For this review, take the finished solid that the model builds, in its own axes (mm). A direction names the side the tool comes from. Round coordinates to 2 decimals unless told otherwise and drop trailing zeros. Loops run counter-clockwise (first coordinate to the right, second up) from the corner with the lowest first, then second, coordinate; pieces in that order, holes last. Notation, with made-up numbers: M 75.5,6 L 112.5,6 A19 ccw 112.5,34 Z; hole C 76,0 d2. An arc over 180 degrees is marked long. Write item = value, one per line. Start each with the question number.
```python
from build123d import *

# Parameters (mm, degrees)
SKETCH1_W           = 118.75
SKETCH1_H           = 24
BOSS_EXTRUDE1_DEPTH = 10
SKETCH2_W           = 3.3
SKETCH2_H           = 9.8
BOSS_EXTRUDE2_DEPTH = 118.75
SKETCH3_W           = 3.3
SKETCH3_H           = 33.8
BOSS_EXTRUDE3_DEPTH = 4.9
CUT_EXTRUDE1_REACH  = 123.333
SKETCH4_R           = 1.9
LPATTERN1_COUNT     = 5
LPATTERN1_PITCH     = 23.75


with BuildPart() as part:
    # Sketch1 → Boss-Extrude1 (new body)
    with BuildSketch(Plane.YZ):
        with Locations((59.375, 12)):
            Rectangle(SKETCH1_W, SKETCH1_H)
    extrude(amount=-BOSS_EXTRUDE1_DEPTH)

    # Sketch2 → Boss-Extrude2 (add, through all)
    with BuildSketch(Plane.XZ):
        with Locations((-5, -4.9)):
            Rectangle(SKETCH2_W, SKETCH2_H)
    extrude(amount=-BOSS_EXTRUDE2_DEPTH)

    # Sketch3 → Boss-Extrude3 (add)
    with BuildSketch(Plane.XZ):
        with Locations((-5, 7.1)):
            Rectangle(SKETCH3_W, SKETCH3_H)
    extrude(amount=BOSS_EXTRUDE3_DEPTH)

    # Sketch4 → Cut-Extrude1 (cut, up to next)
    with BuildSketch(Plane(origin=(-6.65, 0, 0), x_dir=(0, -1, 0), z_dir=(-1, 0, 0)), mode=Mode.PRIVATE) as cut_extrude1_sk1:
        with Locations(Location((-106.875, -5, 0), (0, 0, 90))):
            Circle(SKETCH4_R)
    cut_extrude1_tool1 = extrude(cut_extrude1_sk1.sketch, amount=-CUT_EXTRUDE1_REACH, mode=Mode.PRIVATE) & part.part
    cut_extrude1 = cut_extrude1_tool1.solids().sort_by_distance((-6.65, 106.875, -5))[0]
    add(cut_extrude1, mode=Mode.SUBTRACT)

    # LPattern1: Cut-Extrude1 ×5
    with Locations(*[(0, -i * LPATTERN1_PITCH, 0) for i in range(1, LPATTERN1_COUNT)]):
        add(cut_extrude1, mode=Mode.SUBTRACT)


solid = part.part
```
(1) Draft analysis for pull direction Z (two halves, no side actions). For faces 6 (the flat face through (-2, 59, 0)), 7 (the flat face through (-6.65, 52.6, -0.5)), 8 (the cylindrical face through (-5.02, 105.02, -5.41)), state which applies: +Z half, -Z half, draft (parallel to the pull), parting line (faces both ways), or undercut.
(2) Add section D-D on x = -2.25. Write out the cut boundary in (y, z), and give its area (3 significant figures).
(3) Wall thickness on L1, parallel to Y at x = -4.35, z = -5 (3 decimals); L2, parallel to Y at x = -6.5, z = -6.5; L3, parallel to Z at x = -0.5, y = 88: over which ranges is each line inside the solid? List them lowest first.
(4) Add section B-B on y = 91. Write out the cut boundary in (x, z), and give its area (3 significant figures).
(5) Tool access review of faces 1 (the flat face through (-2, 0, 12)), 2 (the flat face through (-8, 0, 12)), 3 (the flat face through (-8, 59, 0)), 4 (the cylindrical face through (-5, 35.7, -6.9)), 5 (the flat face through (-10, 59, 12)): name each direction out of +Z, -Z, +X, -X, +Y, -Y from which nothing blocks a thin tool from reaching the whole face with its end or side.
(6) For pin 1 Ø1.7 at (x, y) = (-8, 83) entering from -Z; pin 2 Ø5 at (y, z) = (106.875, -5) entering from +X; pin 3 Ø1 at (x, z) = (-1.5, 14.5) entering from -Y, all flat-tipped, find the tip position at first contact; note any pin that passes through.
(7) Add section C-C on z = 8. Write out the cut boundary in (x, y).
(8) Add section A-A on z = -5. Write out the cut boundary in (x, y) (3 decimals), and give its area (3 significant figures).
Answer sheet:
q1.face_6 = -Z half
q1.face_7 = draft
q1.face_8 = undercut
q2.outline = M 0,0 L 118.75,0 L 118.75,24 L 0,24 Z
q2.area = 2,850 mm²
q3.L1 = -4.9 to 9.975, 13.775 to 33.725, 37.525 to 57.475, 61.275 to 81.225, 85.025 to 104.975, 108.775 to 118.75
q3.L2 = -4.9 to 10.71, 13.04 to 34.46, 36.79 to 58.21, 60.54 to 81.96, 84.29 to 105.71, 108.04 to 118.75
q3.L3 = 0 to 24
q4.outline = M -10,0 L -6.65,0 L -6.65,-9.8 L -3.35,-9.8 L -3.35,0 L 0,0 L 0,24 L -10,24 Z
q4.area = 272 mm²
q5.face_1 = +Z, -Z, +X, -Y
q5.face_2 = +Z, -Z, -X, -Y
q5.face_3 = -Z, -X, +Y, -Y
q5.face_4 = +X, -X
q5.face_5 = +Z, -Z, -X, +Y, -Y
q6.pin_1 = 0
q6.pin_2 = -3.35
q6.pin_3 = 0
q7.outline = M -10,0 L -6.65,0 L -6.65,-4.9 L -3.35,-4.9 L -3.35,0 L 0,0 L 0,118.75 L -10,118.75 Z
q8.outline = M -6.65,-4.9 L -3.35,-4.9 L -3.35,9.975 L -6.65,9.975 Z; M -6.65,13.775 L -3.35,13.775 L -3.35,33.725 L -6.65,33.725 Z; M -6.65,37.525 L -3.35,37.525 L -3.35,57.475 L -6.65,57.475 Z; M -6.65,61.275 L -3.35,61.275 L -3.35,81.225 L -6.65,81.225 Z; M -6.65,85.025 L -3.35,85.025 L -3.35,104.975 L -6.65,104.975 Z; M -6.65,108.775 L -3.35,108.775 L -3.35,118.75 L -6.65,118.75 Z
q8.area = 345 mm²
